```python
from build123d import *

# Parameters (mm, degrees)
SKETCH1_R           = 10
BOSS_EXTRUDE1_DEPTH = 6


with BuildPart() as part:
    # Sketch1 → Boss-Extrude1 (new body)
    with BuildSketch(Plane.XY):
        Polygon((78, 0), (78, -6), (66, -6), (66, 0), (54, 0), (54, -6), (42, -6), (42, 0), (30, 0), (30, -6), (18, -6), (18, 0), (6, 0), (6, -6), (-6, -6), (-6, 0), (-18, 0), (-18, -6), (-30, -6), (-30, 0), (-42, 0), (-42, -6), (-54, -6), (-54, 0), (-66, 0), (-66, -6), (-78, -6), (-78, 0), (-87.5, 0), (-87.5, 14.5), (-93.5, 14.5), (-93.5, 26.5), (-87.5, 26.5), (-87.5, 38.5), (-93.5, 38.5), (-93.5, 50.5), (-87.5, 50.5), (-87.5, 62.5), (-93.5, 62.5), (-93.5, 74.5), (-87.5, 74.5), (-87.5, 86.5), (-93.5, 86.5), (-93.5, 98.5), (-87.5, 98.5), (-87.5, 110.5), (-93.5, 110.5), (-93.5, 122.5), (-87.5, 122.5), (-87.5, 134.5), (-93.5, 134.5), (-93.5, 146.5), (-87.5, 146.5), (-87.5, 158.5), (-93.5, 158.5), (-93.5, 170.5), (-87.5, 170.5), (-87.5, 182.5), (-93.5, 182.5), (-93.5, 194.5), (-87.5, 194.5), (-87.5, 206.5), (-93.5, 206.5), (-93.5, 218.5), (-87.5, 218.5), (-87.5, 230.5), (-93.5, 230.5), (-93.5, 242.5), (-87.5, 242.5), (-87.5, 254.5), (-93.5, 254.5), (-93.5, 266.5), (-87.5, 266.5), (-87.5, 278.5), (-93.5, 278.5), (-93.5, 290.5), (-87.5, 290.5), (-87.5, 305), (-78, 305), (-78, 311), (-66, 311), (-66, 305), (-54, 305), (-54, 311), (-42, 311), (-42, 305), (-30, 305), (-30, 311), (-18, 311), (-18, 305), (-6, 305), (-6, 311), (6, 311), (6, 305), (18, 305), (18, 311), (30, 311), (30, 305), (42, 305), (42, 311), (54, 311), (54, 305), (66, 305), (66, 311), (78, 311), (78, 305), (87.5, 305), (87.5, 290.5), (93.5, 290.5), (93.5, 278.5), (87.5, 278.5), (87.5, 266.5), (93.5, 266.5), (93.5, 254.5), (87.5, 254.5), (87.5, 242.5), (93.5, 242.5), (93.5, 230.5), (87.5, 230.5), (87.5, 218.5), (93.5, 218.5), (93.5, 206.5), (87.5, 206.5), (87.5, 194.5), (93.5, 194.5), (93.5, 182.5), (87.5, 182.5), (87.5, 170.5), (93.5, 170.5), (93.5, 158.5), (87.5, 158.5), (87.5, 146.5), (93.5, 146.5), (93.5, 134.5), (87.5, 134.5), (87.5, 122.5), (93.5, 122.5), (93.5, 110.5), (87.5, 110.5), (87.5, 98.5), (93.5, 98.5), (93.5, 86.5), (87.5, 86.5), (87.5, 74.5), (93.5, 74.5), (93.5, 62.5), (87.5, 62.5), (87.5, 50.5), (93.5, 50.5), (93.5, 38.5), (87.5, 38.5), (87.5, 26.5), (93.5, 26.5), (93.5, 14.5), (87.5, 14.5), (87.5, 0), align=None)
        with Locations((33.5, 54)):
            Circle(SKETCH1_R, mode=Mode.SUBTRACT)
    extrude(amount=BOSS_EXTRUDE1_DEPTH)


solid = part.part
```
For this review, take the finished solid that the model builds, in its own axes (mm). A direction names the side the tool comes from. Round coordinates to 2 decimals unless told otherwise and drop trailing zeros. Loops run counter-clockwise (first coordinate to the right, second up) from the corner with the lowest first, then second, coordinate; pieces in that order, holes last.
Q1. Machinability: for faces 1 (the face through (-91, 290.5, 3)), 2 (the face through (1, 155, 6)), 3 (the face through (91, 110.5, 3)), 4 (the face through (-66, 308, 3)), 5 (the face through (-87.5, 80, 3)), which of the approach directions +Z, -Z, +X, -X, +Y, -Y give a long, thin tool a straight path to every point of the face, cutting with its end or side? Answer none if there is none.
Result sheet:
face 1: +Z, -Z, -X, +Y
face 2: +Z, +X, -X, +Y, -Y
face 3: +Z, -Z, +X
face 4: +Z, -Z, +Y
face 5: +Z, -Z, -X
Q2. To check wall thickness, follow line 1 along Y through (x, z) = (33.5, 3.8); line 2 along Y through (x, z) = (-7, 2.05); line 3 along X through (y, z) = (153, 2.75). State the ranges of each line that lie inside material, in increasing order.
Result sheet:
line 1: y = 0 to 44, 64 to 305
line 2: y = 0 to 305
line 3: x = -87.5 to 87.5
Q3. Mouldability with a two-part tool opening along Y and no side actions: class faces 6 (the face through (6, 308, 3)), 7 (the face through (24, 311, 3)), 8 (the face through (-91, 26.5, 3)), 9 (the face through (-90, 278.5, 3)) as +Y half, -Y half, draft (parallel to the pull), parting line (faces both ways), or undercut.
Result sheet:
face 6: draft
face 7: +Y half
face 8: undercut
face 9: undercut
Q4. Add section B-B on y = 54. Write out the cut boundary in (x, z), plus the area to 3 significant figures.
Result sheet:
outline: (-87.5, 0) - (23.5, 0) - (23.5, 6) - (-87.5, 6) - close; (43.5, 0) - (87.5, 0) - (87.5, 6) - (43.5, 6) - close
area: 930 mm2
Q5. Add section A-A on x = 38.5. Write out the cut boundary in (y, z).
Result sheet:
outline: (0, 0) - (45.34, 0) - (45.34, 6) - (0, 6) - close; (62.66, 0) - (305, 0) - (305, 6) - (62.66, 6) - close
Q6. Insertion check: pin 1 Ø1.8 at (y, z) = (-4, 1.5) entering from -X; pin 2 Ø1.8 at (y, z) = (-4, 4.5) entering from +X; pin 3 Ø1.8 at (x, z) = (-91, 3.5) entering from +Y; pin 4 Ø5 at (x, y) = (0.5, 63) entering from -Z. Each pin has a flat end and moves straight along its axis. Give the tip position at first contact, or say it passes through.
Result sheet:
pin 1: stops at x = -78
pin 2: stops at x = 78
pin 3: stops at y = 290.5
pin 4: stops at z = 0
Q7. Add section C-C on x = 12. Write out the cut boundary in (y, z).
Result sheet:
outline: (0, 0) - (305, 0) - (305, 6) - (0, 6) - close
